Could you check a few things on this model? Use its own coordinates, in mm. Face numbers are marked on the shaded views. A direction names the side the tool comes from. Give positions to 0.01 mm unless a question says otherwise; leave off trailing zeros. Write each loop counter-clockwise with the first axis right and the second up, starting at its lowest first coordinate (ties: lowest second). Pieces come first, ordered by that corner, then holes. Notation, with made-up numbers: (83.5, 49.25) - (137.5, 49.25) arc R12 ccw to (137.5, 53.25) - close; hole circle Ø3 at (56.25, 67.5). An arc over 180 degrees is marked (long way). Write item = value, one per line.
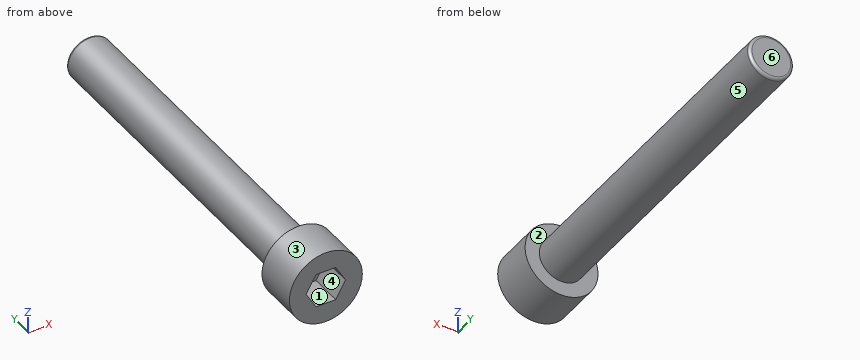
from build123d import *

# Parameters (mm, degrees)
SKETCH1_R           = 6.4
BOSS_EXTRUDE1_DEPTH = 67.83
SKETCH2_OUTSIDE_W   = 28.84
SKETCH2_OUTSIDE_H   = 28.84
SKETCH2_OUTSIDE_R   = 3.9
CUT_EXTRUDE1_DEPTH  = 60
CUT_EXTRUDE2_DEPTH  = 5.64
FILLET1_R           = 0.5


with BuildPart() as part:
    # Sketch1 → Boss-Extrude1 (new body)
    with BuildSketch(Plane(origin=(0, 0, 0), x_dir=(1, 0, 0), z_dir=(0, 1, 0))):
        Circle(SKETCH1_R)
    extrude(amount=BOSS_EXTRUDE1_DEPTH)

    # Sketch2 outside → Cut-Extrude1 (cut)
    with BuildSketch(Plane(origin=(0, 67.83, 0), x_dir=(1, 0, 0), z_dir=(0, 1, 0))):
        Rectangle(SKETCH2_OUTSIDE_W, SKETCH2_OUTSIDE_H)
        Circle(SKETCH2_OUTSIDE_R, mode=Mode.SUBTRACT)
    extrude(amount=-CUT_EXTRUDE1_DEPTH, mode=Mode.SUBTRACT)

    # Sketch8 → Cut-Extrude2 (cut)
    with BuildSketch(Plane.XZ):
        Polygon((3.464101615, 0), (1.732050808, 3), (-1.732050808, 3), (-3.464101615, 0), (-1.732050808, -3), (1.732050808, -3), align=None)
    extrude(amount=-CUT_EXTRUDE2_DEPTH, mode=Mode.SUBTRACT)

    # Fillet1
    fillet1_edges = [part.edges().sort_by_distance(p)[0] for p in [
        (-3.9, 67.83, 0),
    ]]
    fillet(fillet1_edges, radius=FILLET1_R)


solid = part.part
1. Thinking about a two-plate mould opening in Z: for the marked faces 4, 5 and 6, which applies, pulls with the +Z half, pulls with the -Z half, needs draft (parallel to the pull), parting line crosses it, or undercut?
Filled sheet:
face_4 = undercut
face_5 = parting line crosses it
face_6 = needs draft
2. For pin 1 (2 mm diameter, centred on x = -1.5, y = 32, fed in from -Z); pin 2 (1 mm diameter, centred on x = -1, y = 4, fed in from -Z); pin 3 (4 mm diameter, centred on y = 48.5, z = 3, fed in from -X), each with a flat end and sliding along its axis, tell me the tip position at first contact or that it passes through.
Filled sheet:
pin_1 = -3.87
pin_2 = -6.38
pin_3 = -3.77
3. Which directions (+Z, -Z, +X, -X, +Y, -Y) give clear straight access to the entire face, cutting with the end or side of a thin tool? Please do the marked faces 1, 2 and 3.
Filled sheet:
face_1 = -Y
face_2 = +Y
face_3 = +Y, -Y
4. If we section it at C-C, the plane z = -4.5: Please give me the cut outline in (x, y).
Filled sheet:
outline = (-4.55, 0) - (4.55, 0) - (4.55, 7.83) - (-4.55, 7.83) - close
5. I need wall thicknesses on line 1 (Y direction, x = 4, z = -1.5); line 2 (Y direction, x = -1, z = -1.5); line 3 (X direction, y = 28.5, z = -2.5). Which ranges of each line are inside material? Lowest first, please.
Filled sheet:
line_1 = 0 to 7.83
line_2 = 5.64 to 67.83
line_3 = -2.99 to 2.99
6. If we section it at A-A, the plane x = 0: Please give me the cut outline in (y, z).
Filled sheet:
outline = (0, -6.4) - (7.83, -6.4) - (7.83, -3.9) - (67.33, -3.9) arc R0.5 ccw to (67.83, -3.4) - (67.83, 3.4) arc R0.5 ccw to (67.33, 3.9) - (7.83, 3.9) - (7.83, 6.4) - (0, 6.4) - (0, 3) - (5.64, 3) - (5.64, -3) - (0, -3) - close
7. If we section it at D-D, the plane x = -4.5: Please give me the cut outline in (y, z), and give its area (3 significant figures).
Filled sheet:
outline = (0, -4.55) - (7.83, -4.55) - (7.83, 4.55) - (0, 4.55) - close
area = 71.3 mm2
8. If we section it at B-B, the plane y = 31.5: Please give me the cut outline in (x, z), and give its area (3 significant figures).
Filled sheet:
outline = circle Ø7.8 at (0, 0)
area = 47.8 mm2
